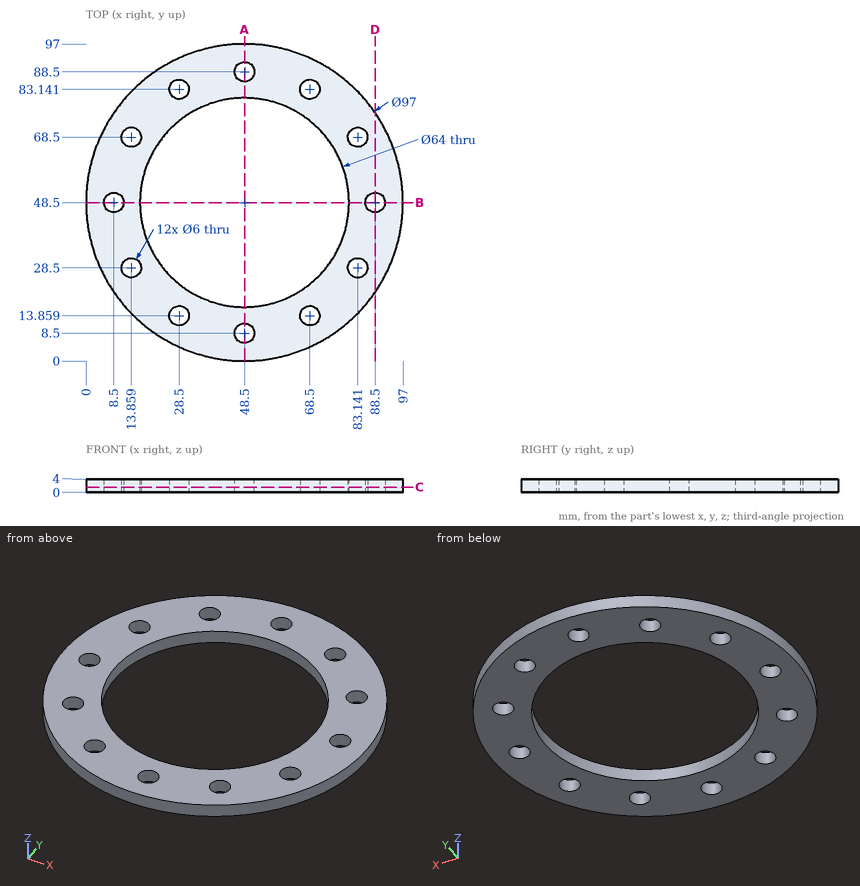
Here's the drawing with two shaded views (mm, measured from the low corner). I have some questions. Round coordinates to 2 decimals unless told otherwise and drop trailing zeros. Loops run counter-clockwise (first coordinate to the right, second up) from the corner with the lowest first, then second, coordinate; pieces in that order, holes last.
Item 1: Suppose I cut it at A-A, the plane x = 48.5. Write out the boundary of the cut face in (y, z).
Item 2: Suppose I cut it at C-C, the plane z = 1.55. State how many separate pieces and enclosed holes the cut face has, then the cut area to 3 significant figures.
Item 3: Will these pins go through, and if not, where does the flat tip stop? pin 1 Ø7 at (x, y) = (8.5, 48.5) entering from -Z; pin 2 Ø5.5 at (x, y) = (28.5, 83.14) entering from -Z.
Item 4: Suppose I cut it at D-D, the plane x = 88.5. Write out the boundary of the cut face in (y, z).
Item 5: Please list where these lines run through material, in increasing order: L1, parallel to X at y = 48, z = 2.3; L2, parallel to Y at x = 27, z = 1.45; L3, parallel to Y at x = 52, z = 0.75.
Reported:
1. outline: (0, 0) - (5.5, 0) - (5.5, 4) - (0, 4) - close; (11.5, 0) - (16.5, 0) - (16.5, 4) - (11.5, 4) - close; (80.5, 0) - (85.5, 0) - (85.5, 4) - (80.5, 4) - close; (91.5, 0) - (97, 0) - (97, 4) - (91.5, 4) - close
2. separate pieces: 1
2. enclosed holes: 13
2. area: 3,830 mm2
3. pin 1: stops at z = 0
3. pin 2: passes through
4. outline: (21.07, 0) - (45.5, 0) - (45.5, 4) - (21.07, 4) - close; (51.5, 0) - (75.93, 0) - (75.93, 4) - (51.5, 4) - close
5. L1: x = 0 to 5.54, 11.46 to 16.5, 80.5 to 85.54, 91.46 to 97
5. L2: y = 5.03 to 11.26, 16.46 to 24.8, 72.2 to 80.54, 85.74 to 91.97
5. L3: y = 0.13 to 16.69, 80.31 to 96.87
